```python
from build123d import *

# Parameters (mm, degrees)
BOSS_EXTRUDE1_DEPTH = 2
SKETCH7_R           = 2.75
CUT_EXTRUDE1_DEPTH  = 104.526033301


with BuildPart() as part:
    # Sketch1 → Boss-Extrude1 (new body)
    with BuildSketch(Plane(origin=(0, 0, 0), x_dir=(1, 0, 0), z_dir=(0, 1, 0))):
        Polygon((-32.806430064, 51.994551896), (60.552740485, 51.994551896), (25.225039266, -83.946442395), (-6.149932227, -83.946442395), (23.249976258, 24.323717363), (-32.806430064, 24.323717363), align=None)
    extrude(amount=BOSS_EXTRUDE1_DEPTH)

    # Sketch7 → Cut-Extrude1 (cut, through all)
    with BuildSketch(Plane(origin=(0, 0, 0), x_dir=(1, 0, 0), z_dir=(0, 1, 0))):
        with Locations(Location((-17.67535185, 46.230759465, 0), (0, 0, 270))):
            Circle(SKETCH7_R)
        with Locations(Location((46.18825301, 18.385111047, 0), (0, 0, 270))):
            Circle(SKETCH7_R)
        with Locations(Location((8.431159892, -54.160966994, 0), (0, 0, 270))):
            Circle(SKETCH7_R)
    extrude(amount=CUT_EXTRUDE1_DEPTH, mode=Mode.SUBTRACT)


solid = part.part
```
The listing builds one solid part. Answer for the finished solid, in the listing's coordinates (mm). A direction names the side the tool comes from. Coordinates: 2 decimals unless noted, no trailing zeros. Order: outer loops, then holes, each group sorted by start corner. A loop starts at its lowest first (then second) coordinate and runs counter-clockwise, first axis right, second up. Notation, with made-up numbers: M -1.5,35.5 L 32.5,35.5 A27 ccw 32.5,67.5 Z; hole C -5,18 d10. An arc over 180 degrees is marked long. Answer as a JSON object with one key per item and string values. Group by question number.
1. Section D-D on z = 34.5 is taken. Write down the section's boundary in (x, y).
2. Section B-B on x = 2.5 is taken. Write down the section's boundary in (y, z).
3. Determine the mould class of faces 1 (the cylindrical face through (9.257, 0.986, 56.784)), 2 (the flat face through (43.136, 0.986, 15.024)), 3 (the flat face through (25, 0, 0)), 4 (the cylindrical face through (-17.554, 0.986, -48.978)) for opening direction X: released by +X, released by -X, zero draft, split by the parting line, or undercut.
4. Flat-ended cylindrical pins translate along their axes: P1, Ø6.5, axis at x = 8.43, z = 54.16, coming from the -Y side; P2, Ø4.5, axis at x = -17.68, z = -46.23, coming from the +Y side; P3, Ø1, axis at x = -7.5, y = 0.5, coming from the +Z side. Find the tip coordinate at first contact, or state that the pin passes through.
5. Straight lines are drawn through the part: line 1 (Z direction, x = -18, y = 0.75); line 2 (Z direction, x = -18.5, y = 0.1); line 3 (Z direction, x = -25, y = 0.95). For each, find the intervals that lie inside material, in ascending order.
6. A tool of negligible diameter and unlimited length cuts with its end or side. For faces 5 (the cylindrical face through (48.915, 0.986, -18.743)), 6 (the flat face through (8.344, 0.986, 30.569)), from which of +Z, -Z, +X, -X, +Y, -Y can it reach the whole face along a straight path? Write none if from no direction.
7. Section C-C on x = -12.5 is taken. Write down the section's boundary in (y, z), then the cut area to 3 significant figures.
8. Section A-A on y = 0.4 is taken. Write down the section's boundary in (x, z), then the cut area to 3 significant figures.
Values follow:
{
 "1": {"outline": "M 7.28,0 L 38.07,0 L 38.07,2 L 7.28,2 Z"},
 "2": {"outline": "M 0,-51.99 L 2,-51.99 L 2,-24.32 L 0,-24.32 Z; M 0,52.09 L 2,52.09 L 2,83.95 L 0,83.95 Z"},
 "3": {"face 1": "undercut", "face 2": "released by +X", "face 3": "zero draft", "face 4": "undercut"},
 "4": {"P1": "y = 0", "P2": "through", "P3": "z = -24.32"},
 "5": {"line 1": "-51.99 to -48.96, -43.5 to -24.32", "line 2": "-51.99 to -48.85, -43.61 to -24.32", "line 3": "-51.99 to -24.32"},
 "6": {"face 5": "+Y, -Y", "face 6": "-X, +Y, -Y"},
 "7": {"outline": "M 0,-51.99 L 2,-51.99 L 2,-24.32 L 0,-24.32 Z", "area": "55.3 mm2"},
 "8": {"outline": "M -32.81,-51.99 L 60.55,-51.99 L 25.23,83.95 L -6.15,83.95 L 23.25,-24.32 L -32.81,-24.32 Z; hole C -17.68,-46.23 d5.5; hole C 8.43,54.16 d5.5; hole C 46.19,-18.39 d5.5", "area": "5,740 mm2"}
}
